from build123d import *

# Parameters (mm, degrees)
BOX130_W                    = 120
BOX130_H                    = 150
BOX130_DEPTH                = 15
BOX130_PITCH_ANGLE          = 36
CYLINDER281_R               = 5
CYLINDER281_DEPTH           = 130
CYLINDER281_PLACEMENT_ANGLE = 126
CYLINDER280_W               = 11
CYLINDER280_H               = 120
CYLINDER280_ANGLE           = 50
CYLINDER280_PLACEMENT_ANGLE = 126
CYLINDER283_R               = 6
CYLINDER283_DEPTH           = 130
CYLINDER283_PLACEMENT_ANGLE = 126
CYLINDER282_W               = 11
CYLINDER282_H               = 120
CYLINDER282_ANGLE           = 90
CYLINDER282_PLACEMENT_ANGLE = 126
CYLINDER279_R               = 11
CYLINDER279_DEPTH           = 120
CYLINDER279_PLACEMENT_ANGLE = 126
CYLINDER278_R               = 20
CYLINDER278_DEPTH           = 120
CYLINDER278_PLACEMENT_ANGLE = 126


with BuildPart() as cubo093:
    # Box130 → Box130 (new body)
    with BuildSketch(Plane.XY):
        with Locations((60, 75)):
            Rectangle(BOX130_W, BOX130_H)
    extrude(amount=BOX130_DEPTH)


with BuildPart() as cubo093_1:
    # Box130 pitch: moved
    add(cubo093.part.rotate(Axis((0, 0, 0), (0, 1, 0)), BOX130_PITCH_ANGLE))


with BuildPart() as cubo093_2:
    # Box130 placement: moved
    add(cubo093_1.part.moved(Location((-296, 17, 92.9))))


with BuildPart() as cilindro168:
    # Cylinder281 → Cylinder281 (new body)
    with BuildSketch(Plane.XY):
        Circle(CYLINDER281_R)
    extrude(amount=CYLINDER281_DEPTH)


with BuildPart() as cilindro168_1:
    # Cylinder281 placement: moved
    add(cilindro168.part.moved(Location((-292, 0, 98.9))).rotate(Axis((-292, 0, 98.9), (0, 1, 0)), CYLINDER281_PLACEMENT_ANGLE))


with BuildPart() as cut298:
    # Cylinder280 → Cylinder280 (revolve)
    with BuildSketch(Plane.XZ):
        with Locations((5.5, 60)):
            Rectangle(CYLINDER280_W, CYLINDER280_H)
    revolve(axis=Axis((0, 0, 0), (0, 0, 1)), revolution_arc=CYLINDER280_ANGLE)


with BuildPart() as cut298_1:
    # Cylinder280 placement: moved
    add(cut298.part.moved(Location((-292, 0, 98.9))).rotate(Axis((-292, 0, 98.9), (0, 1, 0)), CYLINDER280_PLACEMENT_ANGLE))

    # Cut298: cut Cilindro168
    add(cilindro168_1.part, mode=Mode.SUBTRACT)


with BuildPart() as cilindro170:
    # Cylinder283 → Cylinder283 (new body)
    with BuildSketch(Plane.XY):
        Circle(CYLINDER283_R)
    extrude(amount=CYLINDER283_DEPTH)


with BuildPart() as cilindro170_1:
    # Cylinder283 placement: moved
    add(cilindro170.part.moved(Location((-292, 0, 98.9))).rotate(Axis((-292, 0, 98.9), (0, 1, 0)), CYLINDER283_PLACEMENT_ANGLE))


with BuildPart() as cut300:
    # Cylinder282 → Cylinder282 (revolve)
    with BuildSketch(Plane.XZ):
        with Locations((5.5, 60)):
            Rectangle(CYLINDER282_W, CYLINDER282_H)
    revolve(axis=Axis((0, 0, 0), (0, 0, 1)), revolution_arc=CYLINDER282_ANGLE)


with BuildPart() as cut300_1:
    # Cylinder282 placement: moved
    add(cut300.part.moved(Location((-292, 0, 98.9))).rotate(Axis((-292, 0, 98.9), (0, 1, 0)), CYLINDER282_PLACEMENT_ANGLE))

    # Cut299: cut Cilindro170
    add(cilindro170_1.part, mode=Mode.SUBTRACT)

    # Cut300: cut Cut298
    add(cut298_1.part, mode=Mode.SUBTRACT)


with BuildPart() as cilindro166:
    # Cylinder279 → Cylinder279 (new body)
    with BuildSketch(Plane.XY):
        Circle(CYLINDER279_R)
    extrude(amount=CYLINDER279_DEPTH)


with BuildPart() as cilindro166_1:
    # Cylinder279 placement: moved
    add(cilindro166.part.moved(Location((-292, 0, 98.9))).rotate(Axis((-292, 0, 98.9), (0, 1, 0)), CYLINDER279_PLACEMENT_ANGLE))


with BuildPart() as fusion079:
    # Cylinder278 → Cylinder278 (new body)
    with BuildSketch(Plane.XY):
        Circle(CYLINDER278_R)
    extrude(amount=CYLINDER278_DEPTH)


with BuildPart() as fusion079_1:
    # Cylinder278 placement: moved
    add(fusion079.part.moved(Location((-292, 0, 98.9))).rotate(Axis((-292, 0, 98.9), (0, 1, 0)), CYLINDER278_PLACEMENT_ANGLE))

    # Cut297: cut Cilindro166
    add(cilindro166_1.part, mode=Mode.SUBTRACT)

    # Fusion078: union Cut300
    add(cut300_1.part)

    # Fusion079: union Cubo093
    add(cubo093_2.part)


with BuildPart() as fusion079_2:
    # Fusion079 placement: moved
    add(fusion079_1.part.moved(Location((-524, 0, -105))))


solid = fusion079_2.part
The model under review builds one solid part; all positions refer to its coordinate system, in mm. A direction names the side the tool comes from. Give positions to 0.01 mm unless a question says otherwise; leave off trailing zeros. Write each loop counter-clockwise with the first axis right and the second up, starting at its lowest first coordinate (ties: lowest second). Pieces come first, ordered by that corner, then holes.
1. For P1, Ø5, axis at y = 82, z = -47.5, coming from the +X side; P2, Ø5, axis at y = 34.5, z = -7.5, coming from the +X side; P3, Ø3, axis at x = -766, y = 114, coming from the -Z side, all flat-tipped, find the tip position at first contact; note any pin that passes through.
2. Draft analysis for pull direction Z (two halves, no side actions). For faces 1 (the flat face through (-818.45, 9.17, -9.47)), 2 (the cylindrical face through (-769.361, 5.628, -42.556)), 3 (the flat face through (-772.1, 93, -46.9)), state which applies: +Z half, -Z half, draft (parallel to the pull), parting line (faces both ways), or undercut.
3. Add section A-A, the plane y = 80.5. Write out the cut boundary in (x, z), plus the area to 3 significant figures.
4. Wall thickness on L1, parallel to X at y = 4, z = -32.5; L2, parallel to Y at x = -731, z = -77.5; L3, parallel to Z at x = -780, y = 3.5: over which ranges is each line inside the solid? List them lowest first.
5. Tool access review of faces 4 (the flat face through (-769.978, 6.485, -46.263)), 5 (the flat face through (-718.57, 90.95, -76.65)), 6 (the flat face through (-763.32, 93.05, -34.74)): name each direction out of +Z, -Z, +X, -X, +Y, -Y from which nothing blocks a thin tool from reaching the whole face with its end or side.
Worked answers:
1. P1: stops at x = -742.32
1. P2: stops at x = -797.37
1. P3: stops at z = -52.42
2. face 1: +Z half
2. face 2: undercut
2. face 3: -Z half
3. outline: (-820, -12.1) - (-722.92, -82.63) - (-714.1, -70.5) - (-811.18, 0.04) - close
3. area: 1,800 mm2
4. L1: x = -813 to -797.1, -762.23 to -746.32
4. L2: y = -18.42 to -7.75, 7.75 to 18.42
4. L3: z = -56.6 to -45.15, -19.37 to -7.92
5. face 4: none
5. face 5: -Z, +X, +Y, -Y
5. face 6: +Z, +X, +Y
